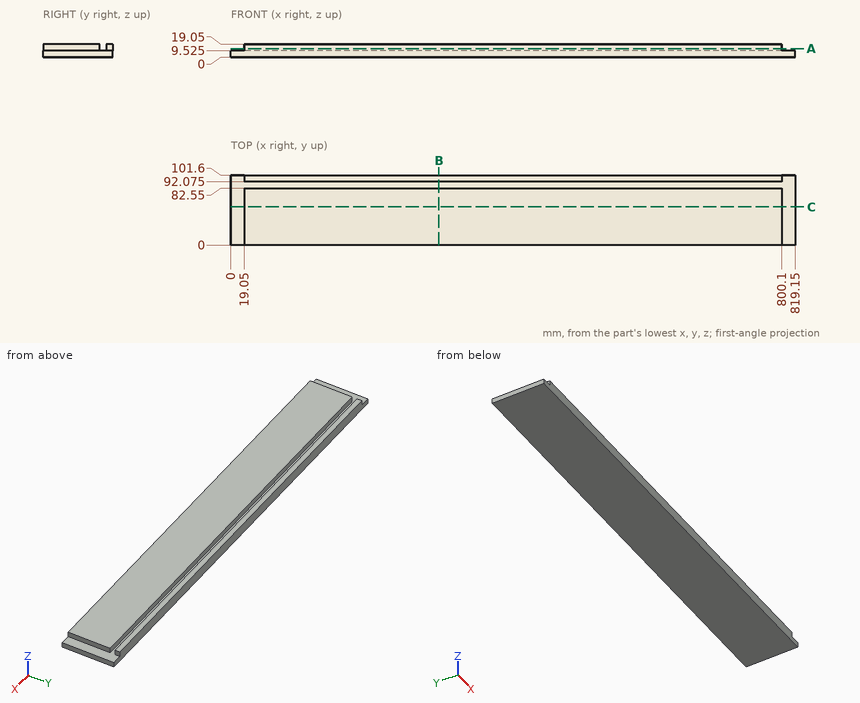
Geometry: see drawing. Coordinates: mm, zero at the bounding-box minimum. Give positions to 0.01 mm unless a question says otherwise; leave off trailing zeros. Order: outer loops, then holes, each group sorted by start corner. A loop starts at its lowest first (then second) coordinate and runs counter-clockwise, first axis right, second up. Notation, with made-up numbers: (-39.75, 65) - (-12.75, 65) arc R19 cw to (-12.75, 71) - close; hole circle Ø1 at (-7, -22.5). An arc over 180 degrees is marked (long way). Use a Markdown table: item, result.
(1) Pin query (flat end, axial travel): pin 1 (1.5 mm diameter, centred on x = 403, y = 26.5, fed in from -Z); pin 2 (1.5 mm diameter, centred on y = 76.5, z = 16, fed in from -X); pin 3 (5 mm diameter, centred on y = 40, z = 16, fed in from +X). Return the tip coordinate at first contact, or that it passes through.
Computed values:
| item | result |
|---|---|
| pin 1 | stops at z = 0 |
| pin 2 | stops at x = 19.05 |
| pin 3 | stops at x = 800.1 |
(2) Section query C-C (y = 55.5). Output: boundary loops of the cut face in (x, z) (3 decimals).
Computed values:
| item | result |
|---|---|
| outline | (0, 0) - (819.15, 0) - (819.15, 9.525) - (800.1, 9.525) - (800.1, 19.05) - (19.05, 19.05) - (19.05, 9.525) - (0, 9.525) - close |
(3) Section query A-A (z = 12.5). Output: boundary loops of the cut face in (x, y) (3 decimals), then the cut area to 3 significant figures.
Computed values:
| item | result |
|---|---|
| outline | (19.05, 0) - (800.1, 0) - (800.1, 82.55) - (19.05, 82.55) - close; (19.05, 92.075) - (800.1, 92.075) - (800.1, 101.6) - (19.05, 101.6) - close |
| area | 71,900 mm2 |
(4) Line query: line 1 (Y direction, x = 585, z = 11) (3 decimals); line 2 (X direction, y = 32, z = 14); line 3 (Z direction, x = 609, y = 92) (3 decimals). Output: solid intervals per line, ascending. Write a range as from..to.
Computed values:
| item | result |
|---|---|
| line 1 | y = 0..82.55, 92.075..101.6 |
| line 2 | x = 19.05..800.1 |
| line 3 | z = 0..9.525 |
(5) Section query B-B (x = 302). Output: boundary loops of the cut face in (y, z) (3 decimals).
Computed values:
| item | result |
|---|---|
| outline | (0, 0) - (101.6, 0) - (101.6, 19.05) - (92.075, 19.05) - (92.075, 9.525) - (82.55, 9.525) - (82.55, 19.05) - (0, 19.05) - close |
